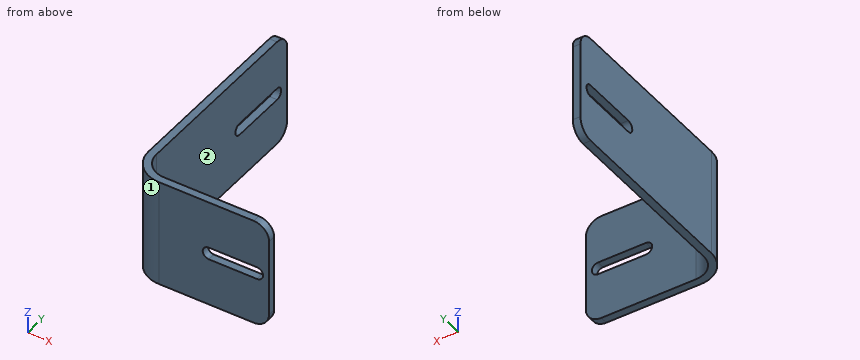
from build123d import *

# Parameters (mm, degrees)
EXTRUDE_THIN1_DEPTH = 35.56
FILLET1_R           = 5.08
CUT_EXTRUDE1_DEPTH  = 71.199112173
CUT_EXTRUDE2_DEPTH  = 92.762357485


with BuildPart() as part:
    # Sketch1 → Extrude-Thin1 (new body)
    with BuildSketch(Plane.XY):
        with BuildLine():
            Line((0, 41.918998188), (0, -23.169286538))
            ThreePointArc((0, -23.169286538), (2.157439192, -28.377805495), (7.365958148, -30.535244686))
            Line((7.365958148, -30.535244686), (43.660042841, -30.535244686))
            Line((43.660042841, -30.535244686), (43.660042841, -33.075244686))
            Line((43.660042841, -33.075244686), (7.365958148, -33.075244686))
            ThreePointArc((7.365958148, -33.075244686), (0.361387967, -30.173856719), (-2.54, -23.169286538))
            Line((-2.54, -23.169286538), (-2.54, 41.918998188))
            Line((-2.54, 41.918998188), (0, 41.918998188))
        make_face()
    extrude(amount=EXTRUDE_THIN1_DEPTH)

    # Fillet1
    fillet1_edges = [part.edges().sort_by_distance(p)[0] for p in [
        (-1.27, 41.918998188, 35.56),
        (-1.27, 41.918998188, 0),
        (43.660042841, -31.805244686, 35.56),
        (43.660042841, -31.805244686, 0),
    ]]
    fillet(fillet1_edges, radius=FILLET1_R)

    # Sketch2 → Cut-Extrude1 (cut, through all)
    with BuildSketch(Plane(origin=(0, 0, 0), x_dir=(0, 0, -1), z_dir=(1, 0, 0))):
        with BuildLine():
            Line((-15.353557986, 36.934347618), (-15.353557986, 18.119499612))
            ThreePointArc((-15.353557986, 18.119499612), (-17.317745415, 16.155312183), (-19.281932844, 18.119499612))
            Line((-19.281932844, 18.119499612), (-19.281932844, 36.934347618))
            ThreePointArc((-19.281932844, 36.934347618), (-17.317745415, 38.898535047), (-15.353557986, 36.934347618))
        make_face()
    extrude(amount=-CUT_EXTRUDE1_DEPTH, mode=Mode.SUBTRACT)

    # Sketch3 → Cut-Extrude2 (cut, through all)
    with BuildSketch(Plane(origin=(0, -30.535244686, 0), x_dir=(1, 0, 0), z_dir=(0, 1, 0))):
        with BuildLine():
            Line((39.637430097, -19.821656487), (23.84441046, -19.821656487))
            ThreePointArc((23.84441046, -19.821656487), (21.802753973, -17.78), (23.84441046, -15.738343513))
            Line((23.84441046, -15.738343513), (39.637430097, -15.738343513))
            ThreePointArc((39.637430097, -15.738343513), (41.679086584, -17.78), (39.637430097, -19.821656487))
        make_face()
    extrude(amount=-CUT_EXTRUDE2_DEPTH, mode=Mode.SUBTRACT)


solid = part.part
Geometry: final body of the model. Coordinates: model frame, mm. Face numbers are marked on the shaded views. A direction names the side the tool comes from. Round coordinates to 2 decimals unless told otherwise and drop trailing zeros. Order: outer loops, then holes, each group sorted by start corner. A loop starts at its lowest first (then second) coordinate and runs counter-clockwise, first axis right, second up.
Q1. Pin query (flat end, axial travel): pin 1 (2 mm diameter, centred on x = 4, z = 26, fed in from -Y); pin 2 (5 mm diameter, centred on y = -25.5, z = 17.5, fed in from +X); pin 3 (2 mm diameter, centred on x = 24, z = 10.5, fed in from +Y). Return the tip coordinate at first contact, or that it passes through.
Result sheet:
pin 1: stops at y = -32.79
pin 2: stops at x = 1.81
pin 3: stops at y = -30.54
Q2. Section A-A, the plane x = 34. Output: boundary loops of the cut face in (y, z), and give its area (3 significant figures).
Result sheet:
outline: (-33.08, 0) - (-30.54, 0) - (-30.54, 15.74) - (-33.08, 15.74) - close; (-33.08, 19.82) - (-30.54, 19.82) - (-30.54, 35.56) - (-33.08, 35.56) - close
area: 80.0 mm2
Q3. Section C-C, the plane z = 18. Output: boundary loops of the cut face in (x, y).
Result sheet:
outline: (-2.54, -23.17) arc R9.91 ccw to (7.37, -33.08) - (21.81, -33.08) - (21.81, -30.54) - (7.37, -30.54) arc R7.37 cw to (0, -23.17) - (0, 16.28) - (-2.54, 16.28) - close; (-2.54, 38.78) - (0, 38.78) - (0, 41.92) - (-2.54, 41.92) - close; (41.67, -33.08) - (43.66, -33.08) - (43.66, -30.54) - (41.67, -30.54) - close
Q4. Material intervals for probe 1 along X at (y, z) = (30, 25.5); probe 2 along Y at (x, z) = (35.5, 11); probe 3 along Y at (x, z) = (6, 2.5), sorted ascending.
Result sheet:
probe 1: x = -2.54 to 0
probe 2: y = -33.08 to -30.54
probe 3: y = -32.98 to -30.41
Q5. Section D-D, the plane z = 22. Output: boundary loops of the cut face in (x, y), and give its area (3 significant figures).
Result sheet:
outline: (-2.54, -23.17) arc R9.91 ccw to (7.37, -33.08) - (43.66, -33.08) - (43.66, -30.54) - (7.37, -30.54) arc R7.37 cw to (0, -23.17) - (0, 41.92) - (-2.54, 41.92) - close
area: 292 mm2
Q6. Access query for the marked faces 1 and 2. Directions: +Z, -Z, +X, -X, +Y, -Y. A direction counts if a zero-diameter tool reaches every point of the face in a straight line with its end or side. Return the directions, or none.
Result sheet:
face 1: +Z, -Z, -X, -Y
face 2: +Z, -Z, +X, +Y
Q7. Section B-B, the plane y = 35.5. Output: boundary loops of the cut face in (x, z).
Result sheet:
outline: (-2.54, 0) - (0, 0) - (0, 15.35) - (-2.54, 15.35) - close; (-2.54, 19.28) - (0, 19.28) - (0, 35.56) - (-2.54, 35.56) - close
